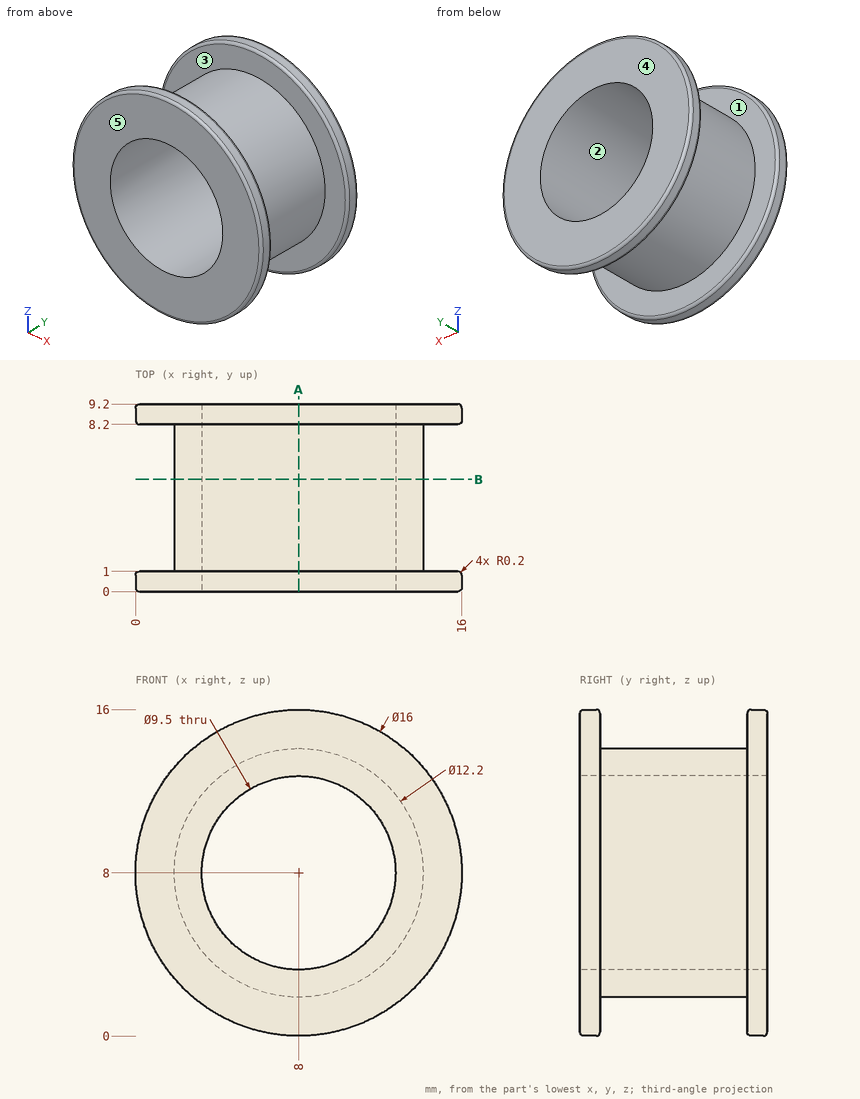
Study the drawing (mm; zero at the part's minimum x, y, z) and answer. A direction names the side the tool comes from. Coordinates: 2 decimals unless noted, no trailing zeros. Loops run counter-clockwise (first coordinate to the right, second up) from the corner with the lowest first, then second, coordinate; pieces in that order, holes last. Notation, with made-up numbers: (45, 67.5) -> (97, 67.5) arc R25 ccw to (97, 87.5) -> close; hole circle Ø2 at (29, 57). An arc over 180 degrees is marked (long way). Answer in a Markdown table with one row per item. Add a question column.
1. The part is cut by section A-A, the plane x = 8. Write down the section's boundary in (y, z).
2. Determine the mould class of the marked faces 3, 4 and 5 for opening direction Y: +Y half, -Y half, draft (parallel to the pull), parting line (faces both ways), or undercut.
3. Consider line 1 (Y direction, x = 5.75, z = 1.5); line 2 (X direction, y = 4.75, z = 8); line 3 (Z direction, x = 6.75, y = 6.75). Determine where each line is inside the solid, lowest interval first. Write a range as [from, to].
4. Flat-ended cylindrical pins translate along their axes: P1, Ø1, axis at y = 3, z = 9, coming from the +X side; P2, Ø1, axis at x = 4, y = 1, coming from the +Z side; P3, Ø1.5, axis at x = 11, y = 5.5, coming from the -Z side. Find the tip coordinate at first contact, or state that the pin passes through.
5. The part is cut by section B-B, the plane y = 5.5. Write down the section's boundary in (x, z).
6. For the marked faces 1 and 2, determine the directions among +Z, -Z, +X, -X, +Y, -Y from which every point of the face is accessible in a straight line to the end or side of a thin tool.
Answer below:
| question | item | result |
|---|---|---|
| 1 | outline | (0, 0.2) arc R0.2 ccw to (0.2, 0) -> (0.8, 0) arc R0.2 ccw to (1, 0.2) -> (1, 1.9) -> (8.2, 1.9) -> (8.2, 0.2) arc R0.2 ccw to (8.4, 0) -> (9, 0) arc R0.2 ccw to (9.2, 0.2) -> (9.2, 3.25) -> (0, 3.25) -> close; (0, 12.75) -> (9.2, 12.75) -> (9.2, 15.8) arc R0.2 ccw to (9, 16) -> (8.4, 16) arc R0.2 ccw to (8.2, 15.8) -> (8.2, 14.1) -> (1, 14.1) -> (1, 15.8) arc R0.2 ccw to (0.8, 16) -> (0.2, 16) arc R0.2 ccw to (0, 15.8) -> close |
| 2 | face 3 | undercut |
| 2 | face 4 | +Y half |
| 2 | face 5 | -Y half |
| 3 | line 1 | [0, 1], [8.2, 9.2] |
| 3 | line 2 | [1.9, 3.25], [12.75, 14.1] |
| 3 | line 3 | [2.03, 3.42], [12.58, 13.97] |
| 4 | P1 | x = 14.08 |
| 4 | P2 | z = 15.18 |
| 4 | P3 | z = 2.33 |
| 5 | outline | circle Ø12.2 at (8, 8); hole circle Ø9.5 at (8, 8) |
| 6 | face 1 | none |
| 6 | face 2 | +Y, -Y |
